```python
from build123d import *

# Parameters (mm, degrees)
SKETCH2_R                               = 45
BOSS_EXTRUDE1_DEPTH                     = 8
SKETCH5_R                               = 23.5
CUT_EXTRUDE1_DEPTH                      = 9
SKETCH6_R                               = 26.9
BOSS_EXTRUDE2_DEPTH                     = 41.148
SKETCH7_R                               = 23.5
CUT_EXTRUDE3_DEPTH                      = 50.148
CBORE_FOR_M8_HEX_HEAD_BOLT1_D           = 6.6
CBORE_FOR_M8_HEX_HEAD_BOLT1_CBORE_D     = 10
CBORE_FOR_M8_HEX_HEAD_BOLT1_CBORE_DEPTH = 5
CIRPATTERN1_COUNT                       = 6


with BuildPart() as part:
    # Sketch2 → Boss-Extrude1 (new body)
    with BuildSketch(Plane.XY):
        Circle(SKETCH2_R)
    extrude(amount=BOSS_EXTRUDE1_DEPTH)

    # Sketch5 → Cut-Extrude1 (cut, through all)
    with BuildSketch(Plane.XY.offset(8)):
        Circle(SKETCH5_R)
    extrude(amount=-CUT_EXTRUDE1_DEPTH, mode=Mode.SUBTRACT)

    # Sketch6 → Boss-Extrude2 (add)
    with BuildSketch(Plane.XY.offset(8)):
        Circle(SKETCH6_R)
    extrude(amount=BOSS_EXTRUDE2_DEPTH)

    # Sketch7 → Cut-Extrude3 (cut, through all)
    with BuildSketch(Plane.XY.offset(49.148)):
        Circle(SKETCH7_R)
    extrude(amount=-CUT_EXTRUDE3_DEPTH, mode=Mode.SUBTRACT)

    # CBORE for M8 Hex Head Bolt1 (through all)
    with Locations(Plane(origin=(0, 32, 0), x_dir=(-1, 0, 0), z_dir=(0, 0, -1))):
        with Locations((0, 0)):
            cbore_for_m8_hex_head_bolt1 = CounterBoreHole(CBORE_FOR_M8_HEX_HEAD_BOLT1_D / 2, CBORE_FOR_M8_HEX_HEAD_BOLT1_CBORE_D / 2, CBORE_FOR_M8_HEX_HEAD_BOLT1_CBORE_DEPTH)

    # CirPattern1: CBORE for M8 Hex Head Bolt1 ×6 about axis
    cirpattern1_axis = Axis((0, 0, 0), (0, 0, 1))
    for i in range(1, CIRPATTERN1_COUNT):
        add(cbore_for_m8_hex_head_bolt1.rotate(cirpattern1_axis, i * 360 / CIRPATTERN1_COUNT), mode=Mode.SUBTRACT)


solid = part.part
```
Geometry check sheet. Reference: the model listing, model coordinates, mm. A direction names the side the tool comes from. Round coordinates to 2 decimals unless told otherwise and drop trailing zeros. Loops run counter-clockwise (first coordinate to the right, second up) from the corner with the lowest first, then second, coordinate; pieces in that order, holes last. Notation, with made-up numbers: (19.5, 51.5) - (56.5, 51.5) arc R8 ccw to (56.5, 66.5) - close; hole circle Ø7 at (-40, -12.5). An arc over 180 degrees is marked (long way). Write item = value, one per line. Start each with the question number.
1. Section check C-C on z = 20.5. Enter the section's corners in (x, y), then the cut area to 3 significant figures.
2. Set-up check for faces 1 (the face through (19, -19, 0)), 2 (the face through (-1.2, -28.7, 5)): record each of +Z, -Z, +X, -X, +Y, -Y from which the full face is reachable in a straight line by a thin tool's end or side.
3. Mould release check, pull along Y, two halves, no side actions. Record for faces 3 (the face through (-25, 13, 5)), 4 (the face through (25.658, 8.08, 28.286)), 5 (the face through (19.4, -19.4, 8)): released by +Y, released by -Y, zero draft, split by the parting line, or undercut.
4. Section check B-B on y = 0. Enter the section's corners in (x, z), then the cut area to 3 significant figures.
5. Section check A-A on x = 0. Enter the section's corners in (y, z), then the cut area to 3 significant figures.
6. Depth check by flat-ended pin: pin 1 (10 mm diameter, centred on y = -18, z = 20.5, fed in from +X); pin 2 (1 mm diameter, centred on y = 21, z = 13, fed in from +X); pin 3 (3 mm diameter, centred on x = -26.5, y = 16, fed in from -Z); pin 4 (3 mm diameter, centred on x = 0.5, y = 29.5, fed in from -Z). Enter the tip coordinate at first touch or a pass-through.
7. Thickness scan on line 1 (Y direction, x = 0, z = 6.65); line 2 (Y direction, x = 15.5, z = 29.5); line 3 (Y direction, x = 20.5, z = 34). Record the ranges inside material, lowest first.
8. Section check D-D on y = 16. Enter the section's corners in (x, z).
Working result:
q1.outline = circle Ø53.8 at (0, 0); hole circle Ø47 at (0, 0)
q1.area = 538 mm^2
q2.face_1 = -Z, +X, -X, +Y, -Y
q2.face_2 = -Z
q3.face_3 = undercut
q3.face_4 = split by the parting line
q3.face_5 = zero draft
q4.outline = (-45, 0) - (-23.5, 0) - (-23.5, 49.15) - (-26.9, 49.15) - (-26.9, 8) - (-45, 8) - close; (23.5, 0) - (45, 0) - (45, 8) - (26.9, 8) - (26.9, 49.15) - (23.5, 49.15) - close
q4.area = 624 mm^2
q5.outline = (-45, 0) - (-37, 0) - (-37, 5) - (-35.3, 5) - (-35.3, 8) - (-45, 8) - close; (-28.7, 5) - (-27, 5) - (-27, 0) - (-23.5, 0) - (-23.5, 49.15) - (-26.9, 49.15) - (-26.9, 8) - (-28.7, 8) - close; (23.5, 0) - (27, 0) - (27, 5) - (28.7, 5) - (28.7, 8) - (26.9, 8) - (26.9, 49.15) - (23.5, 49.15) - close; (35.3, 5) - (37, 5) - (37, 0) - (45, 0) - (45, 8) - (35.3, 8) - close
q5.area = 484 mm^2
q6.pin_1 = 23.55
q6.pin_2 = 17.42
q6.pin_3 = through
q6.pin_4 = 5
q7.line_1 = -45 to -35.3, -28.7 to -23.5, 23.5 to 28.7, 35.3 to 45
q7.line_2 = -21.99 to -17.66, 17.66 to 21.99
q7.line_3 = -17.42 to -11.49, 11.49 to 17.42
q8.outline = (-42.06, 0) - (-32.71, 0) - (-32.71, 5) - (-31.01, 5) - (-31.01, 8) - (-42.06, 8) - close; (-24.41, 5) - (-22.71, 5) - (-22.71, 0) - (-17.21, 0) - (-17.21, 49.15) - (-21.62, 49.15) - (-21.62, 8) - (-24.41, 8) - close; (17.21, 0) - (22.71, 0) - (22.71, 5) - (24.41, 5) - (24.41, 8) - (21.62, 8) - (21.62, 49.15) - (17.21, 49.15) - close; (31.01, 5) - (32.71, 5) - (32.71, 0) - (42.06, 0) - (42.06, 8) - (31.01, 8) - close
